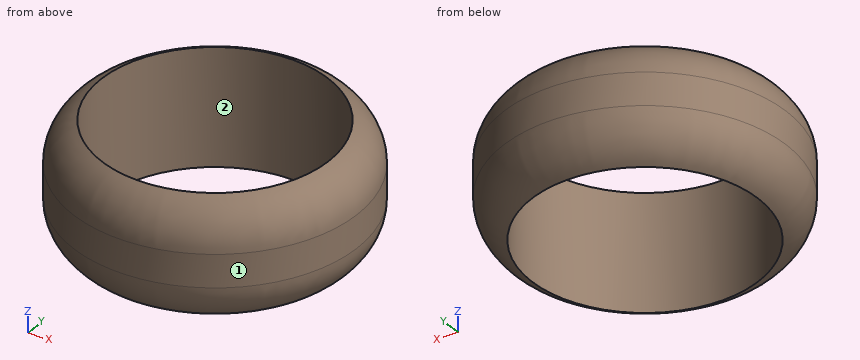
```python
from build123d import *

# Parameters (mm, degrees)
F0_W     = 79.3259590864
F0_H     = 69.0427422523
F2_R     = 25.4
F3_DEPTH = 25.4
F5_D     = 127


with BuildPart() as f1:
    # F0 (on Front) → F1 (revolve)
    with BuildSketch(Plane.XZ):
        with Locations((39.6629795432, 34.5213711262)):
            Rectangle(F0_W, F0_H)
    revolve(axis=Axis((0, 0, 34.5213711262), (0, 0, 1)))

    # F2
    f2_edges = [f1.edges().sort_by_distance(p)[0] for p in [
        (-79.325959, 0, 0),
        (-79.325959, 0, 69.042742),
        (79.325959, 0, 34.521371),
    ]]
    fillet(f2_edges, radius=F2_R)

    # F3 (add): a face of the model
    f3_faces = [f1.faces().sort_by_distance(p)[0] for p in [
        (0, 0, 69.0427422523),
    ]]
    extrude(f3_faces, amount=F3_DEPTH)

    # F5 (through all)
    with Locations(Plane.XY.offset(94.4427422523)):
        with Locations((0, 0)):
            Hole(F5_D / 2)


solid = f1.part
```
Verification items for the finished model (mm, model axes). Face numbers are marked on the shaded views. Round coordinates to 2 decimals unless told otherwise and drop trailing zeros. Order: outer loops, then holes, each group sorted by start corner. A loop starts at its lowest first (then second) coordinate and runs counter-clockwise, first axis right, second up. Notation, with made-up numbers: (79.5, 36) - (131.5, 36) arc R28 cw to (131.5, 61) - close; hole circle Ø8 at (-39.75, 82.25). An arc over 180 degrees is marked (long way). Use CSV: the item, a comma, the result in double quotes. Start each with the question number.
1) Section check D-D, the plane z = 58.5. Record the cut outline in (x, y), plus the area to 3 significant figures.
2) Section check C-C, the plane z = 12.5. Record the cut outline in (x, y).
3) Section check A-A, the plane x = 0. Record the cut outline in (y, z).
4) Thickness scan on L1, parallel to Y at x = 0, z = 30; L2, parallel to Y at x = -26, z = 63; L3, parallel to X at y = 43, z = 46. Record the ranges inside material, lowest first.
5) Mould release check, pull along X, two halves, no side actions. Record for the marked faces 1 and 2: +X half, -X half, draft (parallel to the pull), parting line (faces both ways), or undercut.
6) Go/stop test with flat-tipped pins: P1, Ø3, axis at x = 60, y = 39, coming from the -Z side; P2, Ø3, axis at y = -32, z = 22, coming from the -X side; P3, Ø6, axis at x = -53.5, z = 22, coming from the +Y side; P4, Ø8, axis at x = -38.5, y = -53.5, coming from the +Z side. Record where each tip stops, or that it passes through.
Answers:
1,outline,"circle Ø149.05 at (0, 0); hole circle Ø127 at (0, 0)"
1,area,"4,780 mm²"
2,outline,"circle Ø151.61 at (0, 0); hole circle Ø127 at (0, 0)"
3,outline,"(-79.33, 25.4) arc R25.4 ccw to (-63.5, 1.87) - (-63.5, 67.17) arc R25.4 ccw to (-79.33, 43.64) - close; (63.5, 1.87) arc R25.4 ccw to (79.33, 25.4) - (79.33, 43.64) arc R25.4 ccw to (63.5, 67.17) - close"
4,L1,"y = -79.33 to -63.5, 63.5 to 79.33"
4,L2,"y = -65.39 to -57.93, 57.93 to 65.39"
4,L3,"x = -66.53 to -46.73, 46.73 to 66.53"
5,face 1,"parting line"
5,face 2,"undercut"
6,P1,"stops at z = 5.78"
6,P2,"stops at x = -73.01"
6,P3,"stops at y = 60.92"
6,P4,"stops at z = 67.17"
